Here's the drawing with two shaded views (mm, measured from the low corner). I have some questions. A direction names the side the tool comes from. Give positions to 0.01 mm unless a question says otherwise; leave off trailing zeros. Write each loop counter-clockwise with the first axis right and the second up, starting at its lowest first coordinate (ties: lowest second). Pieces come first, ordered by that corner, then holes. Notation, with made-up numbers: (34, 3.5) -> (44, 3.5) arc R8 cw to (44, 8.5) -> close; hole circle Ø11 at (-16.75, -22). An arc over 180 degrees is marked (long way). One line per item, written item: value.
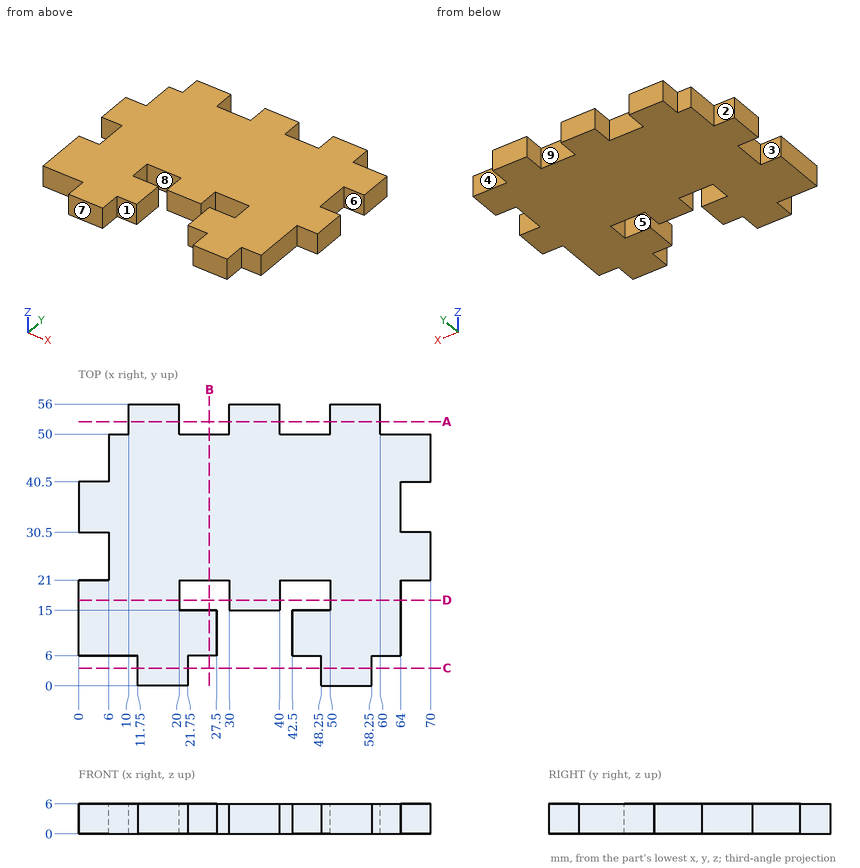
1) If we section it at D-D (y = 17): Write out the boundary of the cut face in (x, z), and give its area (3 significant figures).
Answer list:
outline: (0, 0) -> (20, 0) -> (20, 6) -> (0, 6) -> close; (30, 0) -> (40, 0) -> (40, 6) -> (30, 6) -> close; (50, 0) -> (64, 0) -> (64, 6) -> (50, 6) -> close
area: 264 mm^2
2) I need wall thicknesses on L1, parallel to X at y = 18, z = 2.6; L2, parallel to X at y = 3.5, z = 4.6; L3, parallel to X at y = 11.5, z = 2.25. Which ranges of each line are inside material? Lowest first, please.
Answer list:
L1: x = 0 to 20, 30 to 40, 50 to 64
L2: x = 11.75 to 21.75, 48.25 to 58.25
L3: x = 0 to 27.5, 42.5 to 64
3) Will these pins go through, and if not, where does the flat tip stop? pin 1 (1.8 mm diameter, centred on y = 51.5, z = 2.5, fed in from -X); pin 2 (2 mm diameter, centred on x = 37.5, z = 4, fed in from -Y); pin 3 (1.8 mm diameter, centred on x = 44.5, z = 4.5, fed in from +Y); pin 4 (10 mm diameter, centred on x = 55, y = 16, fed in from -Z).
Answer list:
pin 1: stops at x = 10
pin 2: stops at y = 15
pin 3: stops at y = 50
pin 4: stops at z = 0
4) If we section it at C-C (y = 3.5): Write out the boundary of the cut face in (x, z), and give its area (3 significant figures).
Answer list:
outline: (11.75, 0) -> (21.75, 0) -> (21.75, 6) -> (11.75, 6) -> close; (48.25, 0) -> (58.25, 0) -> (58.25, 6) -> (48.25, 6) -> close
area: 120 mm^2
5) If we section it at B-B (x = 26): Write out the boundary of the cut face in (y, z).
Answer list:
outline: (6, 0) -> (15, 0) -> (15, 6) -> (6, 6) -> close; (21, 0) -> (50, 0) -> (50, 6) -> (21, 6) -> close
6) For the marked faces 1, 2, 3, 4 and 5, which set-ups out of +Z, -Z, +X, -X, +Y, -Y let a thin tool reach every point of the face, with its end or its side?
Answer list:
face 1: +Z, -Z, -Y
face 2: +Z, -Z, -X, +Y
face 3: +Z, -Z, -X
face 4: +Z, -Z, +X, +Y
face 5: +Z, -Z
7) If we section it at A-A (y = 52.5): Write out the boundary of the cut face in (x, z), and give its area (3 significant figures).
Answer list:
outline: (10, 0) -> (20, 0) -> (20, 6) -> (10, 6) -> close; (30, 0) -> (40, 0) -> (40, 6) -> (30, 6) -> close; (50, 0) -> (60, 0) -> (60, 6) -> (50, 6) -> close
area: 180 mm^2
8) We'd pull the mould along Y, two halves only. Please class the marked faces 6, 7, 8 and 9: released by +Y, released by -Y, zero draft, split by the parting line, or undercut.
Answer list:
face 6: undercut
face 7: released by -Y
face 8: undercut
face 9: released by +Y
